Print and shaded views of the part. All mm, measured from the part's lowest x, y and z. Round coordinates to 2 decimals unless told otherwise and drop trailing zeros. Write each loop counter-clockwise with the first axis right and the second up, starting at its lowest first coordinate (ties: lowest second). Pieces come first, ordered by that corner, then holes.
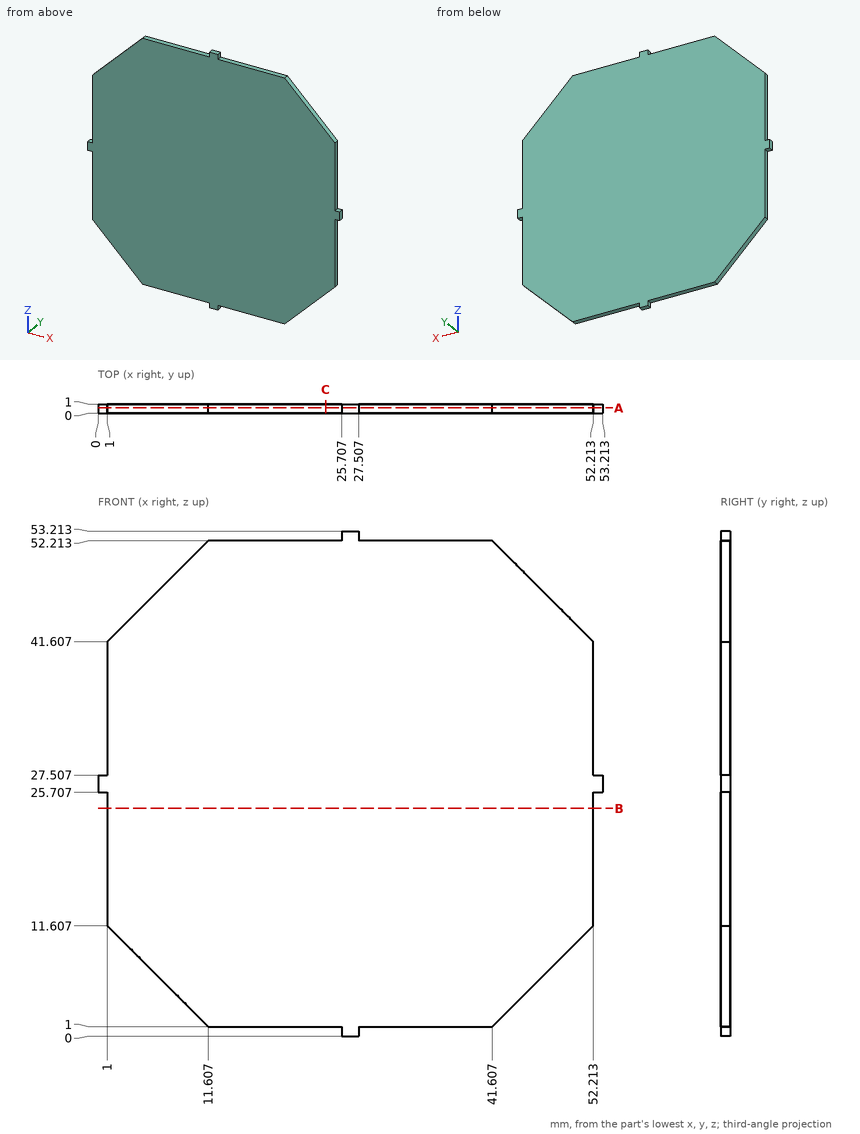
1) Pin check, flat tips, straight feed: pin 1 Ø0.5 at (x, y) = (0.5, 0.5) entering from +Z; pin 2 Ø0.5 at (y, z) = (0.5, 37) entering from +X; pin 3 Ø0.5 at (y, z) = (0.5, 53) entering from +X. Stop position of each tip, or through.
Results:
pin 1: stops at z = 27.51
pin 2: stops at x = 52.21
pin 3: stops at x = 27.51
2) Slice it at C-C (x = 24). Write the cut outline in (y, z).
Results:
outline: (0, 1) - (1, 1) - (1, 52.21) - (0, 52.21) - close
3) Wall check: L1, parallel to X at y = 0.9, z = 39.5; L2, parallel to X at y = 0.25, z = 42.5 (1 decimal). Give the ranges that are in metal, low to high.
Results:
L1: x = 1 to 52.21
L2: x = 1.9 to 51.3
4) Slice it at A-A (y = 0.6). Write the cut outline in (x, z), plus the area to 4 significant figures.
Results:
outline: (0, 25.71) - (1, 25.71) - (1, 11.61) - (11.61, 1) - (25.71, 1) - (25.71, 0) - (27.51, 0) - (27.51, 1) - (41.61, 1) - (52.21, 11.61) - (52.21, 25.71) - (53.21, 25.71) - (53.21, 27.51) - (52.21, 27.51) - (52.21, 41.61) - (41.61, 52.21) - (27.51, 52.21) - (27.51, 53.21) - (25.71, 53.21) - (25.71, 52.21) - (11.61, 52.21) - (1, 41.61) - (1, 27.51) - (0, 27.51) - close
area: 2,405 mm2
5) Slice it at B-B (z = 24). Write the cut outline in (x, y).
Results:
outline: (1, 0) - (52.21, 0) - (52.21, 1) - (1, 1) - close
